The listing builds one solid part. Answer for the finished solid, in the listing's coordinates (mm). Face numbers are marked on the shaded views. Round coordinates to 2 decimals unless told otherwise and drop trailing zeros. Loops run counter-clockwise (first coordinate to the right, second up) from the corner with the lowest first, then second, coordinate; pieces in that order, holes last. Notation, with made-up numbers: (39.5, 41.25) - (92.5, 41.25) arc R10 cw to (92.5, 54.25) - close; hole circle Ø7 at (-38, 88). An arc over 180 degrees is marked (long way). One line per question, with ' | ' between items. Start each with the question number.
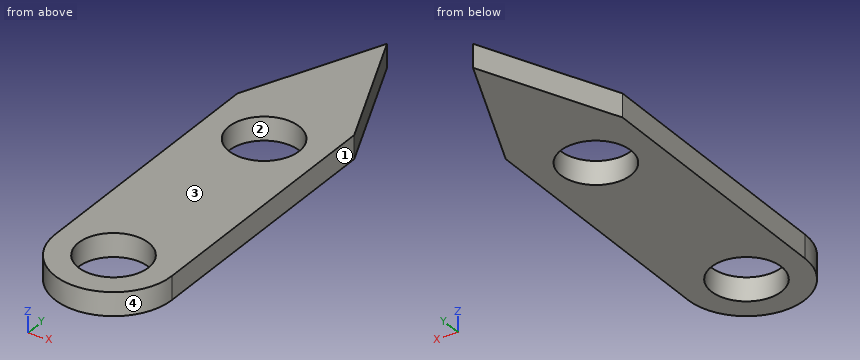
from build123d import *

# Parameters (mm, degrees)
SKETCH_1_R      = 3
EXTRUDE_1_DEPTH = 2


with BuildPart() as part:
    # 草图1 → 凸台-拉伸1 (new body)
    with BuildSketch(Plane.XY):
        with BuildLine():
            Line((4.944222113, 9.446585585), (4.944222113, -9.553414415))
            ThreePointArc((4.944222113, -9.553414415), (-0.055777887, -14.553414415), (-5.055777887, -9.553414415))
            Line((-5.055777887, -9.553414415), (-5.055777887, 9.446585585))
            Line((-5.055777887, 9.446585585), (-5.055777887, 13.446585585))
            Line((-5.055777887, 13.446585585), (-0.055777887, 24.950641748))
            Line((-0.055777887, 24.950641748), (4.944222113, 13.446585585))
            Line((4.944222113, 13.446585585), (4.944222113, 9.446585585))
        make_face()
        with Locations((-0.055777887, 9.446585585)):
            Circle(SKETCH_1_R, mode=Mode.SUBTRACT)
        with Locations((-0.055777887, -9.553414415)):
            Circle(SKETCH_1_R, mode=Mode.SUBTRACT)
    extrude(amount=EXTRUDE_1_DEPTH)


solid = part.part
(1) Find section C-C on z = 0.35. Write down the section's boundary in (x, y), plus the area to 3 significant figures.
(2) This flat-tipped pin is pushed along its axis until it touches: P1, Ø2, axis at x = -2.5, y = -0.5, coming from the -Z side. Where does it stop, or does it pass through?
(3) Find section D-D on y = -7. Write down the section's boundary in (x, z), plus the area to 3 significant figures.
(4) Find section B-B on x = -1.5. Write down the section's boundary in (y, z).
(5) Determine the mould class of the marked faces 1, 2, 3 and 4 for opening direction X: pulls with the +X half, pulls with the -X half, needs draft (parallel to the pull), parting line crosses it, or undercut.
(6) Consider L1, parallel to Y at x = 1.5, z = 1.1; L2, parallel to Y at x = -0.25, z = 1.4; L3, parallel to X at y = 9, z = 1.3. Determine where each line is inside the solid, lowest interval first.
(7) Find section A-A on y = 7. Write down the section's boundary in (x, z).
Answer below:
1) outline: (-5.06, -9.55) arc R5 ccw to (4.94, -9.55) - (4.94, 13.45) - (-0.06, 24.95) - (-5.06, 13.45) - close; hole circle Ø6 at (-0.06, -9.55); hole circle Ø6 at (-0.06, 9.45) | area: 270 mm2
2) P1: z = 0
3) outline: (-5.06, 0) - (-1.63, 0) - (-1.63, 2) - (-5.06, 2) - close; (1.52, 0) - (4.94, 0) - (4.94, 2) - (1.52, 2) - close | area: 13.7 mm2
4) outline: (-14.34, 0) - (-12.18, 0) - (-12.18, 2) - (-14.34, 2) - close; (-6.92, 0) - (6.82, 0) - (6.82, 2) - (-6.92, 2) - close; (12.08, 0) - (21.63, 0) - (21.63, 2) - (12.08, 2) - close
5) face 1: pulls with the +X half | face 2: undercut | face 3: needs draft | face 4: parting line crosses it
6) L1: -14.31 to -12.12, -6.99 to 6.88, 12.01 to 21.37 | L2: -14.55 to -12.55, -6.56 to 6.45, 12.44 to 24.5 | L3: -5.06 to -3.02, 2.91 to 4.94
7) outline: (-5.06, 0) - (-1.79, 0) - (-1.79, 2) - (-5.06, 2) - close; (1.68, 0) - (4.94, 0) - (4.94, 2) - (1.68, 2) - close
